```python
from build123d import *

# Parameters (mm, degrees)
SKETCH043_W             = 21.85
SKETCH043_H             = 12.67
PAD019_DEPTH            = 1.5
PAD020_DEPTH            = 7.42
SKETCH045_R             = 1.65
POCKET018_DEPTH         = 5
SKETCH046_R             = 0.5
POCKET019_DEPTH         = 5
POCKET020_DEPTH         = 6
PAD021_DEPTH            = 5
BODY017_PLACEMENT_ANGLE = 90


with BuildPart() as part:
    # Sketch043 → Pad019 (new body)
    with BuildSketch(Plane.XY):
        with Locations((10.925, 6.335)):
            Rectangle(SKETCH043_W, SKETCH043_H)
    extrude(amount=PAD019_DEPTH)

    # Sketch044 → Pad020 (join)
    with BuildSketch(Plane.XZ.offset(-6.83)):
        with BuildLine():
            Line((6.6, 2.396035), (6.6, 2.996035))
            ThreePointArc((7.79, 3.89207), (7.038545, 3.651836), (6.6, 2.996035))
            Line((7.79, 3.89207), (14.39, 3.89207))
            ThreePointArc((15.58, 2.996035), (15.141455, 3.651836), (14.39, 3.89207))
            Line((15.58, 2.396035), (15.58, 2.996035))
            ThreePointArc((14.39, 1.5), (15.141455, 1.740234), (15.58, 2.396035))
            Line((7.79, 1.5), (14.39, 1.5))
            ThreePointArc((6.6, 2.396035), (7.038545, 1.740234), (7.79, 1.5))
        make_face()
    extrude(amount=-PAD020_DEPTH)

    # Sketch045 → Pocket018 (cut)
    with BuildSketch(Plane.XY):
        with Locations((2.5, 10)):
            Circle(SKETCH045_R)
        with Locations((19.44, 10)):
            Circle(SKETCH045_R)
    extrude(amount=POCKET018_DEPTH, mode=Mode.SUBTRACT)

    # Sketch046 → Pocket019 (cut)
    with BuildSketch(Plane.XY):
        with Locations((4, 1)):
            Circle(SKETCH046_R)
        with Locations((6.54, 1)):
            Circle(SKETCH046_R)
        with Locations((9.08, 1)):
            Circle(SKETCH046_R)
        with Locations((11.62, 1)):
            Circle(SKETCH046_R)
        with Locations((14.16, 1)):
            Circle(SKETCH046_R)
        with Locations((16.7, 1)):
            Circle(SKETCH046_R)
    extrude(amount=POCKET019_DEPTH, mode=Mode.SUBTRACT)

    # Sketch047 → Pocket020 (cut)
    with BuildSketch(Plane.XZ.offset(-9)):
        with BuildLine():
            Line((6.9, 2.402006), (6.9, 3.002006))
            ThreePointArc((7.935662, 3.704011), (7.295255, 3.533843), (6.9, 3.002006))
            Line((7.935662, 3.704011), (14.264338, 3.704011))
            ThreePointArc((15.3, 3.002006), (14.904745, 3.533843), (14.264338, 3.704011))
            Line((15.3, 2.402006), (15.3, 3.002006))
            ThreePointArc((14.264338, 1.7), (14.904745, 1.870168), (15.3, 2.402006))
            Line((7.935662, 1.7), (14.264338, 1.7))
            ThreePointArc((6.9, 2.402006), (7.295255, 1.870168), (7.935662, 1.7))
        make_face()
    extrude(amount=-POCKET020_DEPTH, mode=Mode.SUBTRACT)

    # Sketch048 → Pad021 (join)
    with BuildSketch(Plane.XZ.offset(-9)):
        with BuildLine():
            ThreePointArc((7.9, 2.95), (7.65, 2.7), (7.9, 2.45))
            Line((7.9, 2.45), (14.3, 2.45))
            ThreePointArc((14.3, 2.45), (14.55, 2.7), (14.3, 2.95))
            Line((14.3, 2.95), (7.9, 2.95))
        make_face()
    extrude(amount=-PAD021_DEPTH)


with BuildPart() as part_1:
    # Body017 placement: moved
    add(part.part.moved(Location((28, 11.1, 7))).rotate(Axis((28, 11.1, 7), (0, 0, -1)), BODY017_PLACEMENT_ANGLE))


solid = part_1.part
```
The listing builds one solid part. Answer for the finished solid, in the listing's coordinates (mm). A direction names the side the tool comes from. Coordinates: 2 decimals unless noted, no trailing zeros. Loops run counter-clockwise (first coordinate to the right, second up) from the corner with the lowest first, then second, coordinate; pieces in that order, holes last. Notation, with made-up numbers: (-30, -34.75) -> (15, -34.75) arc R27 cw to (15, 0.25) -> close; hole circle Ø6 at (4, -17). An arc over 180 degrees is marked (long way). Use one line per item in the form item = value. Start each with the question number.
Item 1: A tool of negligible diameter and unlimited length cuts with its end or side. For faces 1 (the face through (39.59, -3.81, 10.53)), 2 (the face through (29.496, 2.085, 7.74)), 3 (the face through (34.83, 0, 10)), from which of +Z, -Z, +X, -X, +Y, -Y can it reach the whole face along a straight path? Write none if from no direction.
Item 2: The part is cut by section A-A on x = 41. Determine the outline of the cut face in (y, z).
Item 3: The mould has two halves that part along Z. Classify faces 4 (the face through (40, 0, 10.704)), 5 (the face through (39.636, -8.125, 7.74)), 6 (the face through (38.49, 4.05, 10.66)), 7 (the face through (37, 0, 9)): released by +Z, released by -Z, zero draft, split by the parting line, or undercut.
Item 4: Flat-ended cylindrical pins translate along their axes: pin 1 Ø0.8 at (y, z) = (1.5, 8) entering from +X; pin 2 Ø5.5 at (x, y) = (38, 8.6) entering from +Z; pin 3 Ø0.6 at (y, z) = (-0.5, 9.5) entering from +X. Find the tip coordinate at first contact, or state that the pin passes through.
Item 5: Consider L1, parallel to Y at x = 38, z = 7.5; L2, parallel to Z at x = 40.75, y = -2.25; L3, parallel to X at y = 2.02, z = 7.5. Determine where each line is inside the solid, lowest interval first. Write a range as [from, to].
Item 6: The part is cut by section D-D on x = 29. Determine the outline of the cut face in (y, z), then the cut area to 3 significant figures.
Item 7: The part is cut by section C-C on x = 37.25. Count the separate pieces of the cut face and the enclosed holes in it, then the cut area to 3 significant figures.
Item 8: The part is cut by section B-B on y = -0.52. Determine the outline of the cut face in (x, z), then the cut area to 3 significant figures.
Answer key:
q1.face_1 = +X
q1.face_2 = +Z, -Z
q1.face_3 = +Z, -X, +Y, -Y
q2.outline = (-4.48, 9.4) arc R1.2 ccw to (-3.29, 8.5) -> (3.31, 8.5) arc R1.2 ccw to (4.5, 9.4) -> (4.5, 10) arc R1.2 ccw to (3.31, 10.89) -> (-3.29, 10.89) arc R1.2 ccw to (-4.48, 10) -> close; (-3.2, 9.45) -> (3.2, 9.45) arc R0.25 ccw to (3.2, 9.95) -> (-3.2, 9.95) arc R0.25 ccw to start; hole (-4.2, 9.4) arc R1 ccw to (-3.16, 8.7) -> (3.16, 8.7) arc R1 ccw to (4.2, 9.4) -> (4.2, 10) arc R1 ccw to (3.16, 10.7) -> (-3.16, 10.7) arc R1 ccw to (-4.2, 10) -> close
q3.face_4 = undercut
q3.face_5 = zero draft
q3.face_6 = released by +Z
q3.face_7 = undercut
q4.pin_1 = 40.67
q4.pin_2 = 8.5
q4.pin_3 = 42
q5.L1 = [-10.75, -9.99], [-6.69, 6.95], [10.25, 11.1]
q5.L2 = [8.5, 8.7], [9.45, 9.95], [10.7, 10.89]
q5.L3 = [28, 28.5], [29.5, 40.67]
q6.outline = (-10.75, 7) -> (-6.1, 7) -> (-6.1, 8.5) -> (-10.75, 8.5) -> close; (-5.1, 7) -> (-3.56, 7) -> (-3.56, 8.5) -> (-5.1, 8.5) -> close; (-2.56, 7) -> (-1.02, 7) -> (-1.02, 8.5) -> (-2.56, 8.5) -> close; (-0.02, 7) -> (1.52, 7) -> (1.52, 8.5) -> (-0.02, 8.5) -> close; (2.52, 7) -> (4.06, 7) -> (4.06, 8.5) -> (2.52, 8.5) -> close; (5.06, 7) -> (6.6, 7) -> (6.6, 8.5) -> (5.06, 8.5) -> close; (7.6, 7) -> (11.1, 7) -> (11.1, 8.5) -> (7.6, 8.5) -> close
q6.area = 23.8 mm2
q7.separate_pieces = 4
q7.enclosed_holes = 1
q7.area = 31.6 mm2
q8.outline = (28, 7) -> (28.5, 7) -> (28.5, 8.5) -> (28, 8.5) -> close; (29.5, 7) -> (40.67, 7) -> (40.67, 8.5) -> (42.25, 8.5) -> (42.25, 8.7) -> (37, 8.7) -> (37, 9.45) -> (42, 9.45) -> (42, 9.95) -> (37, 9.95) -> (37, 10.7) -> (42.25, 10.7) -> (42.25, 10.89) -> (34.83, 10.89) -> (34.83, 8.5) -> (29.5, 8.5) -> close
q8.area = 27.2 mm2
